Can you work these out from the model? Positions are in its coordinate system, mm. Face numbers are marked on the shaded views. A direction names the side the tool comes from. Give positions to 0.01 mm unless a question says otherwise; leave off trailing zeros. Write each loop counter-clockwise with the first axis right and the second up, starting at its lowest first coordinate (ties: lowest second). Pieces come first, ordered by that corner, then holes. Notation, with made-up numbers: (53, 82) -> (61, 82) arc R30 cw to (61, 106) -> close; hole circle Ø3 at (77.25, -36.5). An arc over 180 degrees is marked (long way). Answer as CSV lines item,"result". Start each with the question number.
1. On a 3-axis mill with a long thin cutter (end or side, diameter ignored), from which of +Z, -Z, +X, -X, +Y, -Y can I reach the whole of each face in a straight line? I mean the marked faces 1 and 2. Say none if no direction works.
2. If we section it at B-B on y = -331.5: Write out the boundary of the cut face in (x, z).
3. If we section it at A-A on z = 0: Write out the boundary of the cut face in (x, y), plus the area to 3 significant figures.
4. I'm going to push flat-ended pins straight in: P1, Ø10, axis at x = -44.5, y = -219, coming from the +Z side; P2, Ø6, axis at x = -36, y = -101, coming from the +Z side. Where does each tip first touch, or does it pass through?
5. If we mould it in two halves opening along X, with no side actions, what happens to the marked faces 3, 4 and 5? For each: pulls with the +X half, pulls with the -X half, needs draft (parallel to the pull), parting line crosses it, or undercut.
6. If we section it at C-C on x = -210: Write out the boundary of the cut face in (y, z), plus the area to 3 significant figures.
7. I need wall thicknesses on line 1 (Z direction, x = 0, y = -305); line 2 (Z direction, x = -1.5, y = -276.5); line 3 (X direction, y = -128, z = 65). Which ranges of each line are inside material? Lowest first, please. Write a range as [from, to].
8. If we section it at D-D on y = -219: Write out the boundary of the cut face in (x, z).
```python
from build123d import *

# Parameters (mm, degrees)
F0_W      = 508
F0_H      = 508
F1_DEPTH  = 497.84
F2_R      = 76.2
F3_DEPTH  = 678.243577
F4_SIZE   = 25.4
F6_DEPTH  = 635
F8_DEPTH  = 635
F10_DEPTH = 635
F12_DEPTH = 635
F14_DEPTH = 635
F16_DEPTH = 635


with BuildPart() as f1:
    # F0 (on Front) → F1 (new body)
    with BuildSketch(Plane.XZ):
        Rectangle(F0_W, F0_H)
    extrude(amount=F1_DEPTH)

    # F2 (on face) → F3 (cut, symmetric)
    with BuildSketch(Plane.XZ.offset(497.84)):
        Circle(F2_R)
    extrude(amount=F3_DEPTH, both=True, mode=Mode.SUBTRACT)

    # F4
    f4_edges = [f1.edges().sort_by_distance(p)[0] for p in [
        (-76.2, -497.84, 0),
        (-76.2, 0, 0),
    ]]
    chamfer(f4_edges, length=F4_SIZE)

    # F5 (on Front) → F6 (cut, symmetric)
    with BuildSketch(Plane.XZ):
        Polygon((-206.28102, 269.782053), (-152.4, 215.9), (-98.51898, 269.782053), align=None)
    extrude(amount=F6_DEPTH, both=True, mode=Mode.SUBTRACT)

    # F7 (on Front) → F8 (cut, symmetric)
    with BuildSketch(Plane.XZ):
        Polygon((-53.88102, 269.782053), (0, 215.9), (53.88102, 269.782053), align=None)
    extrude(amount=F8_DEPTH, both=True, mode=Mode.SUBTRACT)

    # F9 (on Front) → F10 (cut, symmetric)
    with BuildSketch(Plane.XZ):
        Polygon((98.51898, 269.782053), (152.4, 215.9), (206.28102, 269.782053), align=None)
    extrude(amount=F10_DEPTH, both=True, mode=Mode.SUBTRACT)

    # F11 (on Right) → F12 (cut, symmetric)
    with BuildSketch(Plane.YZ):
        Polygon((-145.32102, 269.782053), (-91.44, 215.9), (-37.55898, 269.782053), align=None)
    extrude(amount=F12_DEPTH, both=True, mode=Mode.SUBTRACT)

    # F13 (on Right) → F14 (cut, symmetric)
    with BuildSketch(Plane.YZ):
        Polygon((-297.72102, 269.782053), (-243.84, 215.9), (-189.95898, 269.782053), align=None)
    extrude(amount=F14_DEPTH, both=True, mode=Mode.SUBTRACT)

    # F15 (on Right) → F16 (cut, symmetric)
    with BuildSketch(Plane.YZ):
        Polygon((-450.12102, 269.782053), (-396.24, 215.9), (-342.35898, 269.782053), align=None)
    extrude(amount=F16_DEPTH, both=True, mode=Mode.SUBTRACT)


solid = f1.part
```
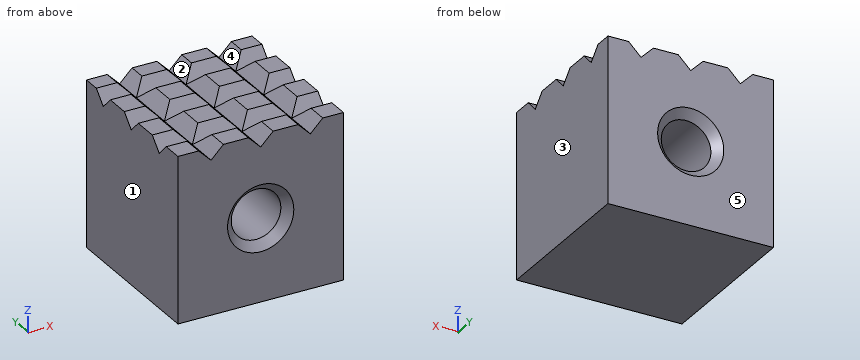
Computed values:
1,face 1,"+Z, -Z, -X, +Y, -Y"
1,face 2,"+Z, +Y, -Y"
2,outline,"(-254, -254) -> (254, -254) -> (254, 254) -> (190.5, 254) -> (152.4, 215.9) -> (114.3, 254) -> (38.1, 254) -> (0, 215.9) -> (-38.1, 254) -> (-114.3, 254) -> (-152.4, 215.9) -> (-190.5, 254) -> (-254, 254) -> close; hole circle Ø152.4 at (0, 0)"
3,outline,"(-254, -497.84) -> (-101.6, -497.84) -> (-76.2, -472.44) -> (-76.2, -25.4) -> (-101.6, 0) -> (-254, 0) -> close; (76.2, -472.44) -> (101.6, -497.84) -> (254, -497.84) -> (254, 0) -> (101.6, 0) -> (76.2, -25.4) -> close"
3,area,"176,000 mm2"
4,P1,"stops at z = 245.74"
4,P2,"stops at z = 228.46"
5,face 3,"pulls with the +X half"
5,face 4,"undercut"
5,face 5,"needs draft"
6,outline,"(-497.84, -254) -> (0, -254) -> (0, 254) -> (-53.34, 254) -> (-91.44, 215.9) -> (-129.54, 254) -> (-205.74, 254) -> (-243.84, 215.9) -> (-281.94, 254) -> (-358.14, 254) -> (-396.24, 215.9) -> (-434.34, 254) -> (-497.84, 254) -> close"
6,area,"249,000 mm2"
7,line 1,"z = [-254, -76.2], [76.2, 215.9]"
7,line 2,"z = [-254, -76.19], [76.19, 217.4]"
7,line 3,"x = [-254, -39.77], [39.77, 254]"
8,outline,"(-254, -254) -> (254, -254) -> (254, 240.74) -> (177.24, 240.74) -> (152.4, 215.9) -> (127.56, 240.74) -> (24.84, 240.74) -> (0, 215.9) -> (-24.84, 240.74) -> (-127.56, 240.74) -> (-152.4, 215.9) -> (-177.24, 240.74) -> (-254, 240.74) -> close; hole circle Ø152.4 at (0, 0)"
